For this review, take the finished solid that the model builds, in its own axes (mm). Face numbers are marked on the shaded views. A direction names the side the tool comes from. Coordinates: 2 decimals unless noted, no trailing zeros. Write each loop counter-clockwise with the first axis right and the second up, starting at its lowest first coordinate (ties: lowest second). Pieces come first, ordered by that corner, then holes.
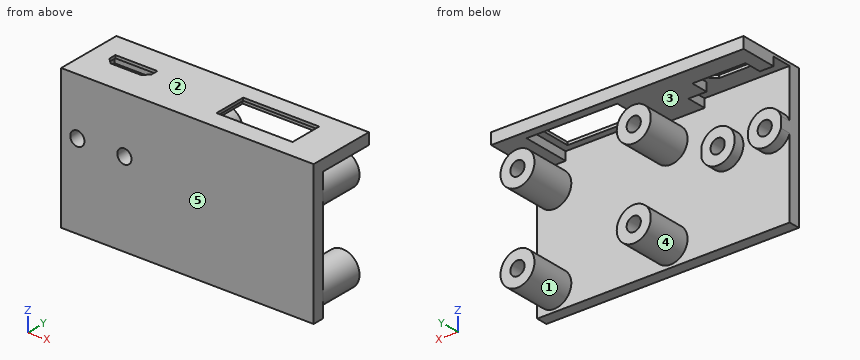
Autodesk Inventor part; units mm, degrees
ref_plane "YZ Plane" through (0, 0, 0) normal (1, 0, 0) x (0, 1, 0)
ref_plane "XZ Plane" through (0, 0, 0) normal (0, 1, 0) x (-1, 0, 0)
ref_plane "XY Plane" through (0, 0, 0) normal (0, 0, 1) x (1, 0, 0)
sketch "Sketch1" plane through (0, 0, 0) normal (0, 1, 0) x (-1, 0, 0)
  line L0 (0, 0) -> (30, 0)
  line L1 (30, 0) -> (30, -25)
  line L2 (30, -25) -> (0, -25)
  line L3 (0, -25) -> (0, 0)
  dimension "d0" = 30
  dimension "d1" = 25
extrude "Extrusion1" add sketch "Sketch1" along normal blind 2
sketch "Sketch2" plane through (0, 2, 0) normal (0, 1, 0) x (1, 0, 0)
  circle A0 centre (-5, 6) radius 3
  circle A1 centre (-5, 21.5) radius 3
  circle A2 centre (-25.5, 6) radius 3
  circle A3 centre (-25.5, 21.5) radius 3
  line L0 (0, 0) -> (0, 25)
  line L1 (0, 25) -> (-30, 25)
  dimension "d4" = 15.5
  dimension "d5" = 15.5
  dimension "d6" = 20.5
  dimension "d7" = 20.5
  dimension "d8" = 0
  dimension "d9" = 0
  dimension "d10" = 6
  dimension "d11" = 6
  dimension "d12" = 6
  dimension "d13" = 6
  dimension "d14" = 5
  dimension "d15" = 3.5
extrude "Extrusion2" add sketch "Sketch2" along normal blind 8
sketch "Sketch3" plane through (-25.5, 10, -6) normal (0, 1, 0) x (1, 0, 0)
  circle A0 centre (20.5, 0) radius 3
  circle A1 centre (20.5, 0) radius 1.25
  circle A2 centre (20.5, 15.5) radius 3
  circle A3 centre (20.5, 15.5) radius 1.25
  circle A4 centre (0, 15.5) radius 3
  circle A5 centre (0, 15.5) radius 1.25
  circle A6 centre (0, 0) radius 3
  circle A7 centre (0, 0) radius 1.25
  point P0 (25.5, -6)
  dimension "d18" = 2.5
  dimension "d19" = 2.5
  dimension "d20" = 2.5
  dimension "d21" = 2.5
extrude "Extrusion3" cut sketch "Sketch3" against normal blind 4 contours A1 | A3 | A5 | A7
sketch "Sketch4" plane through (0, 2, 0) normal (0, 1, 0) x (1, 0, 0)
  line L0 (-30, 25) -> (-30, 0)
  line L1 (0, 0) -> (0, 25)
  line L2 (-30, 0.2) -> (0, 0.2)
  line L3 (0, 0.2) -> (0, 2.2)
  line L4 (0, 2.2) -> (-30, 2.2)
  line L5 (-30, 2.2) -> (-30, 0.2)
  circle A0 centre (-25.5, 6) radius 1.25
  point P0 (0, 0.2)
  dimension "d28" = 5.8
  dimension "d29" = 2
extrude "Extrusion4" add sketch "Sketch4" along normal blind 10 contours L4 L1 L2 L0
sketch "Sketch5" plane through (-30, 2, -0.2) normal (0, 0, 1) x (1, 0, 0)
  line L0 (21.7, 7) -> (8.3, 7)
  line L1 (8.3, 7) -> (8.3, 1.2)
  line L2 (8.3, 1.2) -> (21.7, 1.2)
  line L3 (21.7, 1.2) -> (21.7, 7)
  line L4 (28, 8) -> (22, 8)
  line L5 (0, 0) -> (0, 10)
  point P0 (30, -2)
  point P1 (25, 8)
  dimension "d32" = 13.4
  dimension "d33" = 5.8
  dimension "d36" = 1
  dimension "d37" = 8.3
extrude "Extrusion5" cut sketch "Sketch5" against normal blind 10
sketch "Sketch6" plane through (0, 2, 0) normal (0, 1, 0) x (1, 0, 0)
  line L0 (0, 25) -> (-30, 25)
  line L1 (-30, 0.2) -> (0, 0.2)
  line L2 (-29.3171, 25) -> (-1.9814, 25)
  line L3 (-1.9814, 25) -> (-1.9814, 0.2)
  line L4 (-1.9814, 0.2) -> (-29.3171, 0.2)
  line L5 (-29.3171, 0.2) -> (-29.3171, 25)
  line L6 (-32.5014, 28.1843) -> (1.2029, 28.1843)
  line L7 (1.2029, 28.1843) -> (1.2029, -2.9843)
  line L8 (1.2029, -2.9843) -> (-32.5014, -2.9843)
  line L9 (-32.5014, -2.9843) -> (-32.5014, 28.1843)
  point P0 (-29.3171, 0.2)
extrude "Extrusion6" cut sketch "Sketch6" along normal mid plane 100
sketch "Sketch7" plane through (-1.9814, 2, -2.2) normal (0, 0, -1) x (-1, 0, 0)
  line L0 (0, 0) -> (27.3358, 0)
  line L1 (5.0186, 8.5) -> (21.0186, 8.5)
  line L2 (21.0186, 8.5) -> (21.0186, 0)
  line L3 (21.0186, 0) -> (5.0186, 0)
  line L4 (5.0186, 0) -> (5.0186, 8.5)
  line L5 (6.3186, 1.2) -> (6.3186, 7)
  line L6 (6.3186, 7) -> (19.7186, 7)
  point P0 (-1.9814, -2)
  point P1 (5.0186, 0)
  dimension "d42" = 16
  dimension "d43" = 1.3
  dimension "d44" = 1.5
extrude "Extrusion7" cut sketch "Sketch7" against normal blind 1.5
sketch "Sketch12" plane through (0, 2, 0) normal (0, 1, 0) x (1, 0, 0)
  line L0 (-29.3171, 0.2) -> (-1.9814, 0.2)
  line L1 (-29.3171, 0.2) -> (-46.5, 0.2)
  line L2 (-46.5, 0.2) -> (-46.5, 25)
  line L3 (-46.5, 25) -> (-29.3171, 25)
  line L4 (-29.3171, 25) -> (-29.3171, 0.2)
  circle A0 centre (-25.5, 6) radius 3
  point P0 (0, 0)
  dimension "d49" = 18
extrude "Extrusion8" add sketch "Sketch12" against normal blind 2 contours L1 L2 L3 L4
sketch "Sketch13" plane through (0, 2, 0) normal (0, 1, 0) x (1, 0, 0)
  line L0 (-29.3171, 2.2) -> (-23, 2.2)
  line L1 (-46.5, 25) -> (-46.5, 0.2)
  line L2 (-29.3171, 2.2) -> (-46.5, 2.2)
  line L3 (-46.5, 2.2) -> (-46.5, 0.2)
  line L4 (-46.5, 0.2) -> (-29.3171, 0.2)
  line L5 (-29.3171, 0.2) -> (-29.3171, 2.2)
  point P0 (0, 0)
extrude "Extrusion9" add sketch "Sketch13" along normal up to surface (10 mm away)
sketch "Sketch14" plane through (0, 2, 0) normal (0, 1, 0) x (1, 0, 0)
  line L0 (-46.5, 0.2) -> (-46.5, 25)
  line L1 (-1.9814, 0.2) -> (-46.5, 0.2)
  line L2 (-46.5, 25) -> (-32.5, 25)
  line L3 (-32.5, 25) -> (-32.5, 0.2)
  line L4 (-32.5, 0.2) -> (-46.5, 0.2)
  line L5 (-46.5, 0.2) -> (-46.5, 25)
  circle A0 centre (-35.35, 10.2) radius 3
  arc A1 (-46.5, 9.2633) -> (-46.5, 11.1367) centre (-43.65, 10.2) ccw
  point P0 (0, 0)
  point P1 (-32.5, 9.2633)
  point P2 (-32.5, 11.1367)
  dimension "d54" = 14
  dimension "d55" = 10
  dimension "d56" = 10
  dimension "d57" = 8.3
  dimension "d58" = 6
  dimension "d59" = 6
  dimension "d60" = 2.85
extrude "Extrusion10" add sketch "Sketch14" along normal blind 1.9 contours L0 A1 | A0 L3 picked at (-36.2658, 10.5122)
sketch "Sketch15" plane through (0, 3.9, 0) normal (0, 1, 0) x (1, 0, 0)
  arc A0 (-32.5, 11.1367) -> (-32.5, 9.2633) centre (-35.35, 10.2) ccw
  circle A1 centre (-35.35, 10.2) radius 1.25
  arc A2 (-46.5, 9.2633) -> (-46.5, 11.1367) centre (-43.65, 10.2) ccw
  circle A3 centre (-43.65, 10.2) radius 1.25
  point P0 (0, 0)
  dimension "d63" = 2.5
  dimension "d64" = 2.5
extrude "Extrusion11" cut sketch "Sketch15" against normal blind 4
sketch "Sketch16" plane through (-1.9814, 2, -2.2) normal (0, 0, -1) x (-1, 0, 0)
  line L0 (33.7186, 5.6) -> (41.1186, 5.6)
  line L1 (41.1186, 5.6) -> (41.1186, 4.3)
  line L2 (40.1186, 3.3) -> (34.7186, 3.3)
  line L3 (33.7186, 4.3) -> (33.7186, 5.6)
  line L4 (36.3686, 0) -> (36.3686, 1.9)
  line L5 (36.3686, 1.5842) -> (36.3686, 2.8612)
  line L6 (38.6686, 0) -> (38.6686, 1.9)
  line L7 (38.6686, 1.3572) -> (38.6686, 2.8612)
  line L8 (36.3686, 1.9) -> (30.5186, 1.9)
  line L9 (34.7186, 3.3) -> (40.1186, 3.3)
  line L10 (34.7186, 3.3) -> (33.7186, 4.3)
  line L11 (40.1186, 3.3) -> (41.1186, 4.3)
  point P0 (-1.9814, -2)
  dimension "d68" = 7.4
  dimension "d69" = 2.3
  dimension "d70" = 2.65
  dimension "d71" = 1.4
  dimension "d75" = 1
  dimension "d76" = 1
  dimension "d77" = 135
extrude "Extrusion12" cut sketch "Sketch16" against normal blind 4
sketch "Sketch17" plane through (-1.9814, 2, -2.2) normal (0, 0, -1) x (-1, 0, 0)
  line L0 (0, 0) -> (44.5186, 0)
  line L1 (29.5186, 3.5) -> (44.5186, 3.5)
  line L2 (44.5186, 3.5) -> (44.5186, 0)
  line L3 (44.5186, 0) -> (29.5186, 0)
  line L4 (29.5186, 0) -> (29.5186, 3.5)
  line L5 (36.3686, 1.9) -> (30.5186, 1.9)
  line L6 (36.3686, 1.9) -> (38.6686, 1.9)
  line L7 (38.6686, 0) -> (38.6686, 1.9)
  line L8 (37.5186, 1.9) -> (37.5186, 2.6823)
  line L9 (32.7186, 3.5) -> (42.1186, 3.5)
  line L10 (42.1186, 3.5) -> (42.1186, 6.6)
  line L11 (42.1186, 6.6) -> (32.7186, 6.6)
  line L12 (32.7186, 6.6) -> (32.7186, 3.5)
  line L13 (33.7186, 5.6) -> (41.1186, 5.6)
  line L14 (33.7186, 4.3) -> (33.7186, 5.6)
  line L15 (41.1186, 5.6) -> (41.1186, 4.3)
  point P0 (-1.9814, -2)
  point P1 (29.5186, 0)
  dimension "d80" = 1.6
  dimension "d81" = 8
  dimension "d82" = 1
  dimension "d83" = 1
  dimension "d84" = 1
extrude "Extrusion13" cut sketch "Sketch17" against normal blind 1.5
sketch "Sketch18" plane through (-1.9814, 2, -0.7) normal (0, 0, -1) x (-1, 0, 0)
  point P0 (-1.9814, -2)
properties part number "USB"
Q1. Draft analysis for pull direction X (two halves, no side actions). For the marked faces 1 and 2, state which applies: +X half, -X half, draft (parallel to the pull), parting line (faces both ways), or undercut.
Ans:
face 1: undercut
face 2: draft
Q2. Add section C-C (x = -5). State the section outline as (y, z) points, then the cut area to 3 significant figures.
Ans:
outline: (0, -25) - (2, -25) - (2, -24.5) - (10, -24.5) - (10, -22.75) - (6, -22.75) - (6, -20.25) - (10, -20.25) - (10, -18.5) - (2, -18.5) - (2, -9) - (10, -9) - (10, -7.25) - (6, -7.25) - (6, -4.75) - (10, -4.75) - (10, -3) - (2, -3) - (2, -2.2) - (12, -2.2) - (12, -0.2) - (0, -0.2) - close
area: 146 mm2
Q3. Add section B-B (z = -10.2). State the section outline as (x, y) points.
Ans:
outline: (-46.5, 0) - (-44.9, 0) - (-44.9, 3.9) - (-46.5, 3.9) - close; (-42.4, 0) - (-36.6, 0) - (-36.6, 3.9) - (-38.35, 3.9) - (-38.35, 2) - (-40.65, 2) - (-40.65, 3.9) - (-42.4, 3.9) - close; (-34.1, 0) - (-1.98, 0) - (-1.98, 2) - (-32.5, 2) - (-32.5, 3.9) - (-34.1, 3.9) - close
Q4. For probe 1 along X at (y, z) = (1.95, -10.2); probe 2 along Z at (x, y) = (-35.35, 2.75); probe 3 along X at (y, z) = (8.15, -6), list the stretches that pass through material, from the lowest coordinate up.
Ans:
probe 1: x = -46.5 to -44.9, -42.4 to -36.6, -34.1 to -1.98
probe 2: z = -13.2 to -11.45, -8.95 to -7.2, -0.7 to -0.2
probe 3: x = -28.5 to -26.75, -24.25 to -22.5, -8 to -6.25, -3.75 to -2
Q5. Add section A-A (x = -20). State the section outline as (y, z) points, then the cut area to 4 significant figures.
Ans:
outline: (0, -25) - (2, -25) - (2, -0.7) - (3.2, -0.7) - (3.2, -0.2) - (0, -0.2) - close; (9, -0.7) - (10.5, -0.7) - (10.5, -2.2) - (12, -2.2) - (12, -0.2) - (9, -0.2) - close
area: 53.95 mm2
Q6. Tool access review of the marked faces 3, 4 and 5: name each direction out of +Z, -Z, +X, -X, +Y, -Y from which nothing blocks a thin tool from reaching the whole face with its end or side.
Ans:
face 3: +X, -X, +Y
face 4: +Y
face 5: +Z, -Z, +X, -X, -Y
Q7. Clearance check with flat-ended pins moving along their axes: pin 1 Ø3 at (x, y) = (-21.5, 9.5) entering from -Z; pin 2 Ø0.8 at (x, z) = (-5.5, -5.5) entering from +Y; pin 3 Ø12 at (x, z) = (-16, -18.5) entering from +Y. State where each tip first meets the part, or that it passes through.
Ans:
pin 1: stops at z = -23.16
pin 2: stops at y = 6
pin 3: stops at y = 2
